Design review of the part shown in the three views and the two pictorial views. Dimensions are in mm from the part's minimum x, y and z. A direction names the side the tool comes from. Give positions to 0.01 mm unless a question says otherwise; leave off trailing zeros. Order: outer loops, then holes, each group sorted by start corner. A loop starts at its lowest first (then second) coordinate and runs counter-clockwise, first axis right, second up.
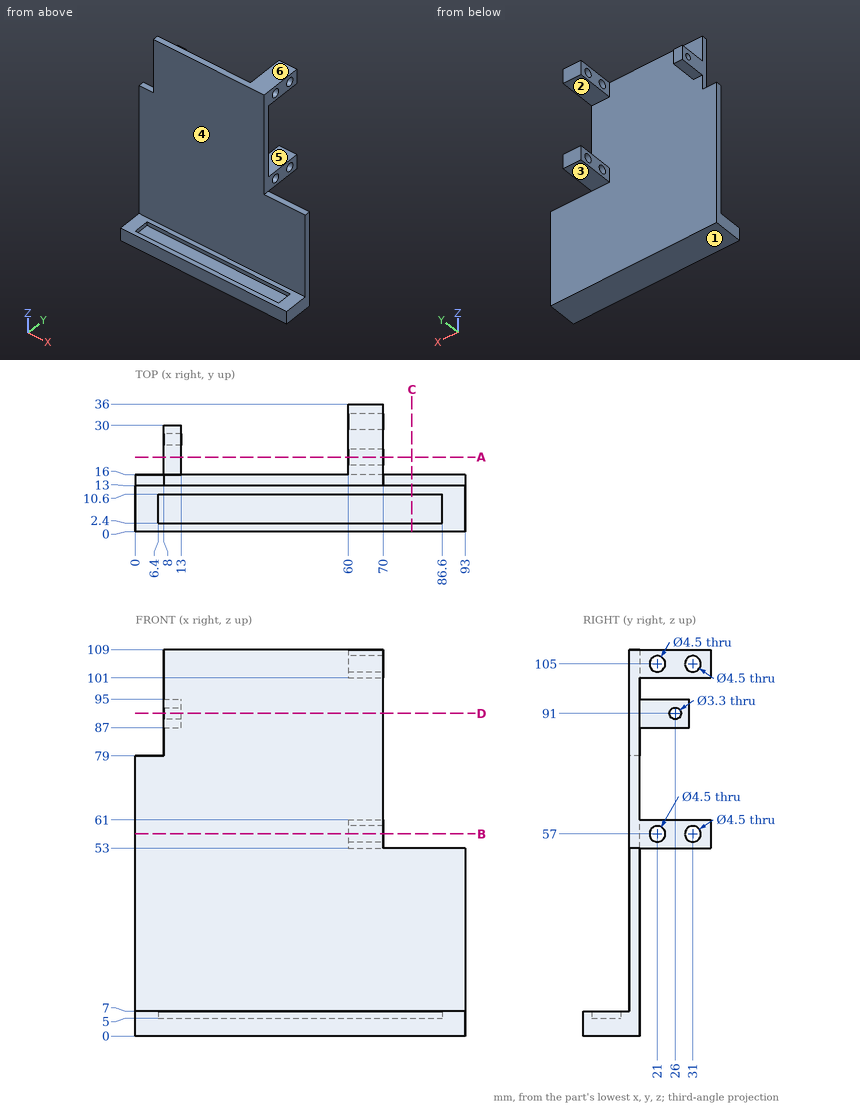
1) Clearance check with flat-ended pins moving along their axes: pin 1 (6.5 mm diameter, centred on y = 26, z = 92, fed in from +X); pin 2 (1 mm diameter, centred on x = 52, z = 6, fed in from +Y); pin 3 (1.5 mm diameter, centred on x = 10, z = 91, fed in from +Y). State where each tip first meets the part, or that it passes through.
Answer sheet:
pin 1: stops at x = 13
pin 2: stops at y = 16
pin 3: stops at y = 30
2) We need section B-B on z = 57. Give the boundary of the cut face in (x, y).
Answer sheet:
outline: (0, 13) - (70, 13) - (70, 18.75) - (60, 18.75) - (60, 16) - (0, 16) - close; (60, 23.25) - (70, 23.25) - (70, 28.75) - (60, 28.75) - close; (60, 33.25) - (70, 33.25) - (70, 36) - (60, 36) - close
3) We need section A-A on y = 21. Give the boundary of the cut face in (x, z), then the cut area to 3 significant figures.
Answer sheet:
outline: (8, 87) - (13, 87) - (13, 95) - (8, 95) - close; (60, 53) - (70, 53) - (70, 54.75) - (60, 54.75) - close; (60, 59.25) - (70, 59.25) - (70, 61) - (60, 61) - close; (60, 101) - (70, 101) - (70, 102.75) - (60, 102.75) - close; (60, 107.25) - (70, 107.25) - (70, 109) - (60, 109) - close
area: 110 mm2
4) We need section D-D on z = 91. Give the boundary of the cut face in (x, y), then the cut area to 4 significant figures.
Answer sheet:
outline: (8, 13) - (70, 13) - (70, 16) - (13, 16) - (13, 24.35) - (8, 24.35) - close; (8, 27.65) - (13, 27.65) - (13, 30) - (8, 30) - close
area: 239.5 mm2
5) We need section C-C on x = 78. Give the boundary of the cut face in (y, z), then the cut area to 3 significant figures.
Answer sheet:
outline: (0, 0) - (16, 0) - (16, 53) - (13, 53) - (13, 7) - (10.6, 7) - (10.6, 5) - (2.4, 5) - (2.4, 7) - (0, 7) - close
area: 234 mm2
6) Draft analysis for pull direction Z (two halves, no side actions). For the marked faces 4, 5 and 6, state which applies: +Z half, -Z half, draft (parallel to the pull), parting line (faces both ways), or undercut.
Answer sheet:
face 4: draft
face 5: undercut
face 6: +Z half
7) Tool access review of the marked faces 1, 2 and 3: name each direction out of +Z, -Z, +X, -X, +Y, -Y from which nothing blocks a thin tool from reaching the whole face with its end or side.
Answer sheet:
face 1: -Z, +X, -X, +Y, -Y
face 2: +X, -X, +Y
face 3: -Z, +X, -X, +Y
8) To check wall thickness, follow line 1 (Y direction, x = 66, z = 105); line 2 (Y direction, x = 61, z = 55.5); line 3 (Z direction, x = 46, y = 12.5). State the ranges of each line that lie inside material, in increasing order.
Answer sheet:
line 1: y = 13 to 18.75, 23.25 to 28.75, 33.25 to 36
line 2: y = 13 to 19.32, 22.68 to 29.32, 32.68 to 36
line 3: z = 0 to 7
